Autodesk Inventor part; units mm, degrees
ref_plane "YZ Plane" through (0, 0, 0) normal (1, 0, 0) x (0, 1, 0)
ref_plane "XZ Plane" through (0, 0, 0) normal (0, 1, 0) x (-1, 0, 0)
ref_plane "XY Plane" through (0, 0, 0) normal (0, 0, 1) x (1, 0, 0)
sketch "Sketch2" plane through (0, 0, 0) normal (0, 0, 1) x (1, 0, 0)
  line L0 (-5.1962, 0) -> (-2.5981, 4.5)
  line L1 (-2.5981, 4.5) -> (2.5981, 4.5)
  line L2 (2.5981, 4.5) -> (5.1962, 0)
  line L3 (5.1962, 0) -> (2.5981, -4.5)
  line L4 (2.5981, -4.5) -> (-2.5981, -4.5)
  line L5 (-2.5981, -4.5) -> (-5.1962, 0)
  point P0 (0, 0)
  point P1 (0, 0)
  dimension "d0" = 9
extrude "Extrusion1" add sketch "Sketch2" along normal blind 2
sketch "Sketch3" plane through (0, 0, 0) normal (0, 1, 0) x (-1, 0, 0)
  line L0 (5.1962, 0) -> (5.1962, 2)
  line L1 (2.5981, 2) -> (-2.5981, 2)
  line L2 (0, 2) -> (1.585, 2)
  line L3 (2.5981, 2) -> (5.1962, 2)
  line L4 (5.1962, 2) -> (4.4462, 2)
  line L5 (1.585, 2) -> (1.585, 2.5)
  line L6 (4.4462, 2) -> (4.4462, 2.5)
  arc A0 (4.4462, 2.5) -> (1.585, 2.5) centre (3.0156, 2.5) ccw
  line L7 (0, 2) -> (0, 5.5151)
  point P0 (0, 0)
  dimension "d3" = 1.585
  dimension "d4" = 0.75
  dimension "d5" = 0.5
  dimension "d6" = 0.5
revolve "Revolution1" add sketch "Sketch3" angle 360 about axis through (0, 0, 2) along (0, 0, 1)
sketch "Sketch4" plane through (0, 0, 2) normal (0, 0, 1) x (1, 0, 0)
  circle A0 centre (0, 0) radius 1.585
  point P0 (0, 0)
extrude "Extrusion2" cut sketch "Sketch4" against normal through all
sketch "Sketch5" plane through (0, 0, 0) normal (0, 0, -1) x (-1, 0, 0)
  circle A0 centre (0, 0) radius 3
  dimension "d10" = 6
extrude "Extrusion3" cut sketch "Sketch5" against normal blind 1.5
properties part number "sealNut" material "Nickel-Copper Alloy 400"
Check sheet for the modelled part. Datum: model origin and axes. Units: mm. A direction names the side the tool comes from. Round coordinates to 2 decimals unless told otherwise and drop trailing zeros. Write each loop counter-clockwise with the first axis right and the second up, starting at its lowest first coordinate (ties: lowest second). Pieces come first, ordered by that corner, then holes. Notation, with made-up numbers: (64, -30.5) - (92, -30.5) arc R15 ccw to (92, -13.5) - close; hole circle Ø1 at (81, -24.5). An arc over 180 degrees is marked (long way). Return JSON: item names as keys, results as strings.
Q1. Cross-section at C-C (z = 3.3). Record the boundary of the cut face in (x, y).
Returned:
{"outline": "circle Ø8.4 at (0, 0); hole circle Ø3.66 at (0, 0)"}
Q2. Draft check along Y on faces 4 (the flat face through (3.915, -2.218, 0.986)), 5 (the flat face through (-1.3, -1.3, 1.5)), 6 (the flat face through (1, 3, 0)). Enter one of: released by +Y, released by -Y, zero draft, split by the parting line, or undercut.
Returned:
{"face 4": "released by -Y", "face 5": "undercut", "face 6": "zero draft"}
Q3. Cross-section at A-A (z = 0.5). Record the boundary of the cut face in (x, y), then the cut area to 3 significant figures.
Returned:
{"outline": "(-5.2, 0) - (-2.6, -4.5) - (2.6, -4.5) - (5.2, 0) - (2.6, 4.5) - (-2.6, 4.5) - close; hole circle Ø6 at (0, 0)", "area": "41.9 mm²"}
Q4. Access from +Z, -Z, +X, -X, +Y, -Y to the whole of each face (thin tool, end or side, straight path). Record for faces 1 (the flat face through (-3.88, -2.28, 0.99)), 2 (the cylindrical face through (3.528, 2.705, 2.254)), 3 (the cylindrical face through (3, 0, 1)).
Returned:
{"face 1": "+Z, -Z, -X, -Y", "face 2": "+Z", "face 3": "-Z"}
Q5. Scan lines: L1, parallel to X at y = 0, z = 2.1 (3 decimals); L2, parallel to Y at x = 0, z = 1.1; L3, parallel to X at y = 0, z = 3.55. Record each from-to range of solid material in increasing order. Write a range as from..to.
Returned:
{"L1": "x = -4.446..-1.585, 1.585..4.446", "L2": "y = -4.5..-3, 3..4.5", "L3": "x = -3.99..-2.04, 2.04..3.99"}
Q6. Depth check by flat-ended pin: P1, Ø3, axis at x = 0, y = 1, coming from the -Z side; P2, Ø5, axis at x = 0, y = 0, coming from the +Z side; P3, Ø2, axis at x = 2, z = 3.5, coming from the -Y side. Enter the tip coordinate at first touch or a pass-through.
Returned:
{"P1": "stops at z = 1.5", "P2": "stops at z = 3.83", "P3": "stops at y = -4.22"}
